from build123d import *


with BuildPart() as f1:
    # F0 (on Front) → F1 (revolve)
    with BuildSketch(Plane.XZ):
        with BuildLine():
            Line((0, 2.169048), (0, 6.169048))
            Line((0, 6.169048), (-21.568638, 6.169048))
            ThreePointArc((-21.568638, 6.169048), (-24.917051, 7.45581), (-26.542019, 10.653794))
            Line((-26.542019, 10.653794), (-40.792739, 148.206101))
            ThreePointArc((-40.792739, 148.206101), (-42.988192, 149.989352), (-44.771443, 147.793899))
            Line((-44.771443, 147.793899), (-29.552598, 0.896949))
            ThreePointArc((-29.552598, 0.896949), (-29.227604, 0.257352), (-28.557922, 0))
            Line((-28.557922, 0), (-24.557922, 0))
            Line((-24.557922, 0), (-21.31824, 2.169048))
            Line((-21.31824, 2.169048), (0, 2.169048))
        make_face()
    revolve(axis=Axis((0, 0, 4.169048), (0, 0, -1)))


solid = f1.part
Could you check a few things on this model? Use its own coordinates, in mm. A direction names the side the tool comes from. Coordinates: 2 decimals unless noted, no trailing zeros. Order: outer loops, then holes, each group sorted by start corner. A loop starts at its lowest first (then second) coordinate and runs counter-clockwise, first axis right, second up. Notation, with made-up numbers: (1.25, 8.5) -> (34.25, 8.5) arc R33 ccw to (34.25, 36.5) -> close; hole circle Ø6 at (58.5, 41). An arc over 180 degrees is marked (long way). One line per question, with ' | ' between items.
Q1. If I drill on L1, parallel to Z at x = -11, y = 11; L2, parallel to Y at x = 7.5, z = 87.5; L3, parallel to Y at x = 14, z = 69.5, over which ranges is the centre line in solid material (lowest first)?
Return value:
L1: 2.17 to 6.17 | L2: -37.79 to -33.68, 33.68 to 37.79 | L3: -33.88 to -29.48, 29.48 to 33.88
Q2. Imagine slicing it at A-A on x = 0. Please give me the cut outline in (y, z), and give its area (3 significant figures).
Return value:
outline: (-44.77, 147.79) -> (-29.55, 0.9) arc R1 ccw to (-28.56, 0) -> (-24.56, 0) -> (-21.32, 2.17) -> (21.32, 2.17) -> (24.56, 0) -> (28.56, 0) arc R1 ccw to (29.55, 0.9) -> (44.77, 147.79) arc R2 ccw to (40.79, 148.21) -> (26.54, 10.65) arc R5 cw to (21.57, 6.17) -> (-21.57, 6.17) arc R5 cw to (-26.54, 10.65) -> (-40.79, 148.21) arc R2 ccw to start | area: 1,430 mm²
Q3. Imagine slicing it at D-D on z = 122.5. Please give me the cut outline in (x, y).
Return value:
outline: circle Ø84.3 at (0, 0); hole circle Ø76.26 at (0, 0)
Q4. I'm going to push flat-ended pins straight in: P1, Ø12, axis at x = -19, y = -27, coming from the -Z side; P2, Ø3, axis at x = -4, z = 55.5, coming from the -Y side; P3, Ø2, axis at y = -34.5, z = 109.5, coming from the -X side; P4, Ø3, axis at y = 9, z = 16, coming from the -X side. Where does each tip first touch, or does it pass through?
Return value:
P1: z = 0 | P2: y = -35.2 | P3: x = -23.31 | P4: x = -30.23
Q5. Imagine slicing it at C-C on z = 67.5. Please give me the cut outline in (x, y), and give its area (3 significant figures).
Return value:
outline: circle Ø72.91 at (0, 0); hole circle Ø64.86 at (0, 0) | area: 870 mm²
Q6. Thinking about a two-plate mould opening in Y: for faces 3 (the face through (29.406, -22.548, 73.317)), 4 (the face through (0, 0, 2.169)), 5 (the face through (-12.6, 21.3, 0)), which applies, pulls with the +Y half, pulls with the -Y half, needs draft (parallel to the pull), parting line crosses it, or undercut?
Return value:
face 3: parting line crosses it | face 4: undercut | face 5: needs draft
Q7. On a 3-axis mill with a long thin cutter (end or side, diameter ignored), from which of +Z, -Z, +X, -X, +Y, -Y can I reach the whole of each face in a straight line? I mean faces 1 (the face through (0, 0, 6.169)), 2 (the face through (-20.484, 6.451, 2.064)). Say none if no direction works.
Return value:
face 1: +Z | face 2: -Z
